```python
from build123d import *

# Parameters (mm, degrees)
F0_W     = 10
F0_H     = 10
F1_DEPTH = 10
F2_SIZE  = 9.99999


# Not quite as in the source:
# - a fillet or chamfer is up to 0.001 mm smaller than in the source, because OpenCascade refuses the exact size


with BuildPart() as f1:
    # F0 (on Top) → F1 (new body)
    with BuildSketch(Plane.XY):
        Rectangle(F0_W, F0_H)
    extrude(amount=F1_DEPTH)

    # F2 (size 10 in the source; OpenCascade refuses exactly that, so slightly less here)
    f2_edges = [f1.edges().sort_by_distance(p)[0] for p in [
        (0, 5, 0),
    ]]
    chamfer(f2_edges, length=F2_SIZE)


solid = f1.part
```
CAD build for the part. Positions are in the model's coordinates, mm. Round coordinates to 2 decimals unless told otherwise and drop trailing zeros. Order: outer loops, then holes, each group sorted by start corner. A loop starts at its lowest first (then second) coordinate and runs counter-clockwise, first axis right, second up.
Q1. Slice it at C-C (z = 1.75). Write the cut outline in (x, y), and give its area (3 significant figures).
Q2. Two-plate mould, pull along X, no slides. Class faces 1 (the flat face through (0, 0, 5)), 2 (the flat face through (-5, -1, 6)), 3 (the flat face through (5, -1, 6)): pulls with the +X half, pulls with the -X half, needs draft (parallel to the pull), parting line crosses it, or undercut.
Q3. Drop flat-ended pins along their axis: pin 1 (1.5 mm diameter, centred on x = -2.5, y = 3, fed in from -Z); pin 2 (1 mm diameter, centred on x = 0.5, z = 9, fed in from +Y); pin 3 (1.5 mm diameter, centred on x = 1, z = 5, fed in from +Y). Give the stop position or say it passes through.
Q4. Wall check: L1, parallel to Y at x = -3.25, z = 9.5; L2, parallel to Z at x = 3.75, y = -2.5; L3, parallel to Z at x = 4.5, y = -3.5. Give the ranges that are in metal, low to high.
Q5. Slice it at B-B (y = -2.5). Write the cut outline in (x, z), and give its area (3 significant figures).
Results below:
1. outline: (-5, -5) - (5, -5) - (5, -3.25) - (-5, -3.25) - close
1. area: 17.5 mm2
2. face 1: needs draft
2. face 2: pulls with the -X half
2. face 3: pulls with the +X half
3. pin 1: stops at z = 7.25
3. pin 2: stops at y = 4.5
3. pin 3: stops at y = 0.75
4. L1: y = -5 to 4.5
4. L2: z = 2.5 to 10
4. L3: z = 1.5 to 10
5. outline: (-5, 2.5) - (5, 2.5) - (5, 10) - (-5, 10) - close
5. area: 75.0 mm2
